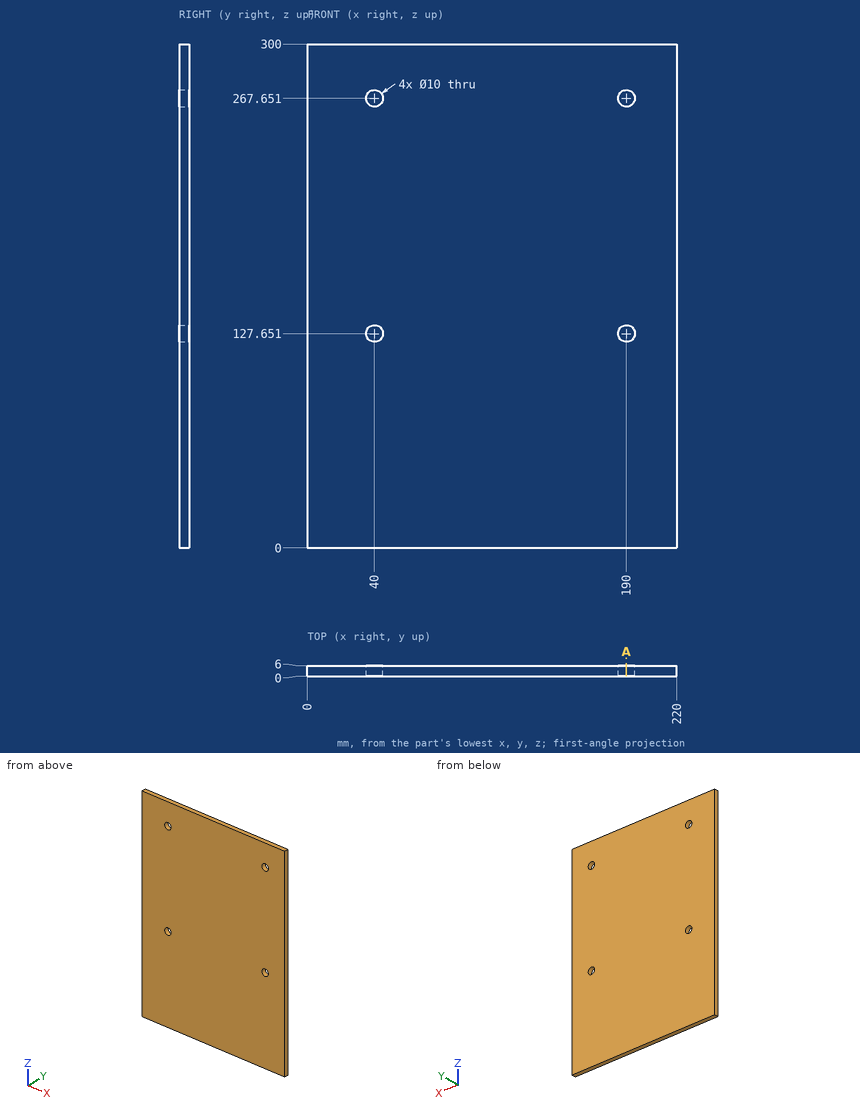
For this review, use the dimensioned drawing (mm, ordinates from the lowest corner) and the shaded views. Give positions to 0.01 mm unless a question says otherwise; leave off trailing zeros. Order: outer loops, then holes, each group sorted by start corner. A loop starts at its lowest first (then second) coordinate and runs counter-clockwise, first axis right, second up. Notation, with made-up numbers: M -20.5,-26 L 36.5,-26 A29 cw 36.5,-3 Z; hole C 7,34 d10. An arc over 180 degrees is marked long. One line per question, with ' | ' between items. Start each with the question number.
1) Clearance check with a flat-ended pin moving along its axis: P1, Ø11.5, axis at x = 190, z = 127.65, coming from the -Y side. State where the tip first meets the part, or that it passes through.
2) Consider section A-A, the plane x = 190. Give the boundary of the cut face in (y, z), then the cut area to 3 significant figures.
3) Wall thickness on L1, parallel to Z at x = 190, y = 4.65; L2, parallel to X at y = 3.75, z = 127.5; L3, parallel to X at y = 2.35, z = 126: over which ranges is each line inside the solid? List them lowest first. Write a range as from..to.
Found:
1) P1: stops at y = 0
2) outline: M 0,0 L 6,0 L 6,122.65 L 0,122.65 Z; M 0,132.65 L 6,132.65 L 6,262.65 L 0,262.65 Z; M 0,272.65 L 6,272.65 L 6,300 L 0,300 Z | area: 1,680 mm²
3) L1: z = 0..122.65, 132.65..262.65, 272.65..300 | L2: x = 0..35, 45..185, 195..220 | L3: x = 0..35.28, 44.72..185.28, 194.72..220
